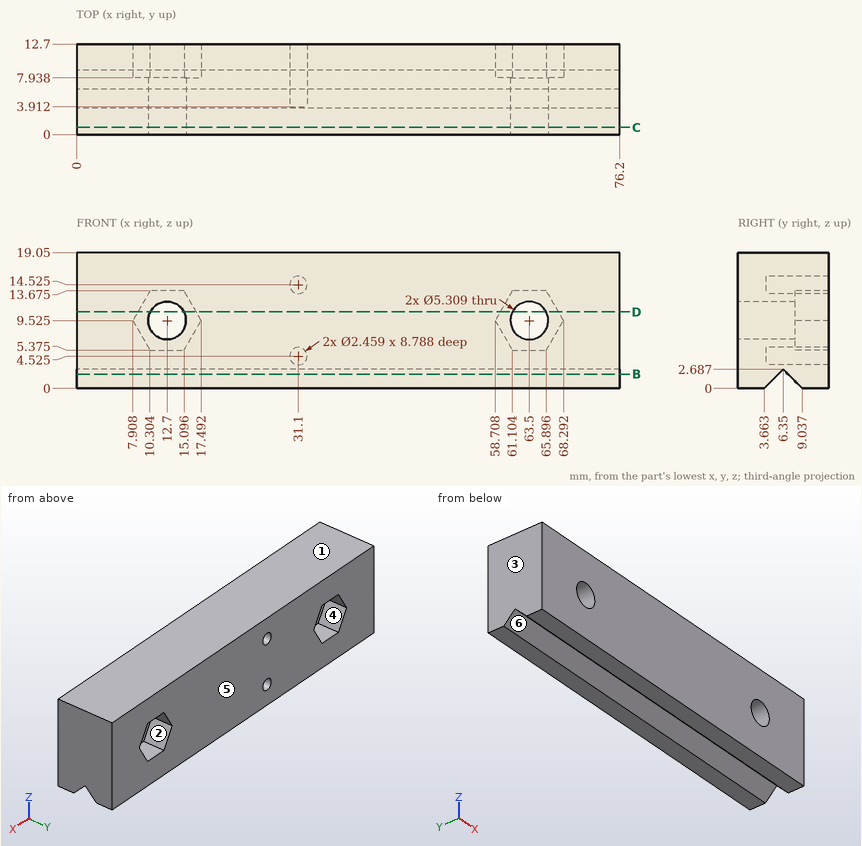
Geometry check sheet. Reference: drawing and pictorial views, mm from the part's lowest x, y, z. A direction names the side the tool comes from. Give positions to 0.01 mm unless a question says otherwise; leave off trailing zeros. Loops run counter-clockwise (first coordinate to the right, second up) from the corner with the lowest first, then second, coordinate; pieces in that order, holes last. Notation, with made-up numbers: M -34.5,18 L 15.5,18 A23 cw 15.5,49 Z; hole C -18,-33.5 d4. An arc over 180 degrees is marked long. One line per question, with ' | ' between items.
Item 1: Section check D-D, the plane z = 10.75. Record the cut outline in (x, y) (1 decimal), plus the area to 3 significant figures.
Completed:
outline: M 0,0 L 10.3,0 L 10.3,7.9 L 8.6,7.9 L 8.6,12.7 L 0,12.7 Z; M 15.1,0 L 61.1,0 L 61.1,7.9 L 59.4,7.9 L 59.4,12.7 L 16.8,12.7 L 16.8,7.9 L 15.1,7.9 Z; M 65.9,0 L 76.2,0 L 76.2,12.7 L 67.6,12.7 L 67.6,7.9 L 65.9,7.9 Z | area: 815 mm^2
Item 2: Thickness scan on line 1 (X direction, y = 3.25, z = 9.25); line 2 (Z direction, x = 31, y = 9.25); line 3 (X direction, y = 7.75, z = 14.5). Record the ranges inside material, lowest first. Write a range as [from, to].
Completed:
line 1: x = [0, 10.06], [15.34, 60.86], [66.14, 76.2] | line 2: z = [0, 3.3], [5.75, 13.3], [15.75, 19.05] | line 3: x = [0, 29.87], [32.33, 76.2]
Item 3: Section check B-B, the plane z = 2. Record the cut outline in (x, y).
Completed:
outline: M 0,0 L 76.2,0 L 76.2,5.66 L 0,5.66 Z; M 0,7.04 L 76.2,7.04 L 76.2,12.7 L 0,12.7 Z
Item 4: Depth check by flat-ended pin: P1, Ø4, axis at x = 64, z = 7.5, coming from the +Y side; P2, Ø2, axis at x = 31.1, z = 4.525, coming from the +Y side. Enter the tip coordinate at first touch or a pass-through.
Completed:
P1: stops at y = 7.94 | P2: stops at y = 3.91
Item 5: Draft check along X on the marked faces 1, 2, 3 and 4. Enter one of: +X half, -X half, draft (parallel to the pull), parting line (faces both ways), or undercut.
Completed:
face 1: draft | face 2: undercut | face 3: -X half | face 4: undercut
Item 6: Tool access check on the marked faces 5 and 6. Record the directions out of +Z, -Z, +X, -X, +Y, -Y that give a thin tool (end or side, any length) a straight path to the whole face; none if there is none.
Completed:
face 5: +Z, -Z, +X, -X, +Y | face 6: -Z, +X, -X
Item 7: Section check C-C, the plane y = 1. State how many separate pieces and enclosed holes the cut face has, plus the area to 3 significant figures.
Completed:
separate pieces: 1 | enclosed holes: 2 | area: 1,410 mm^2
